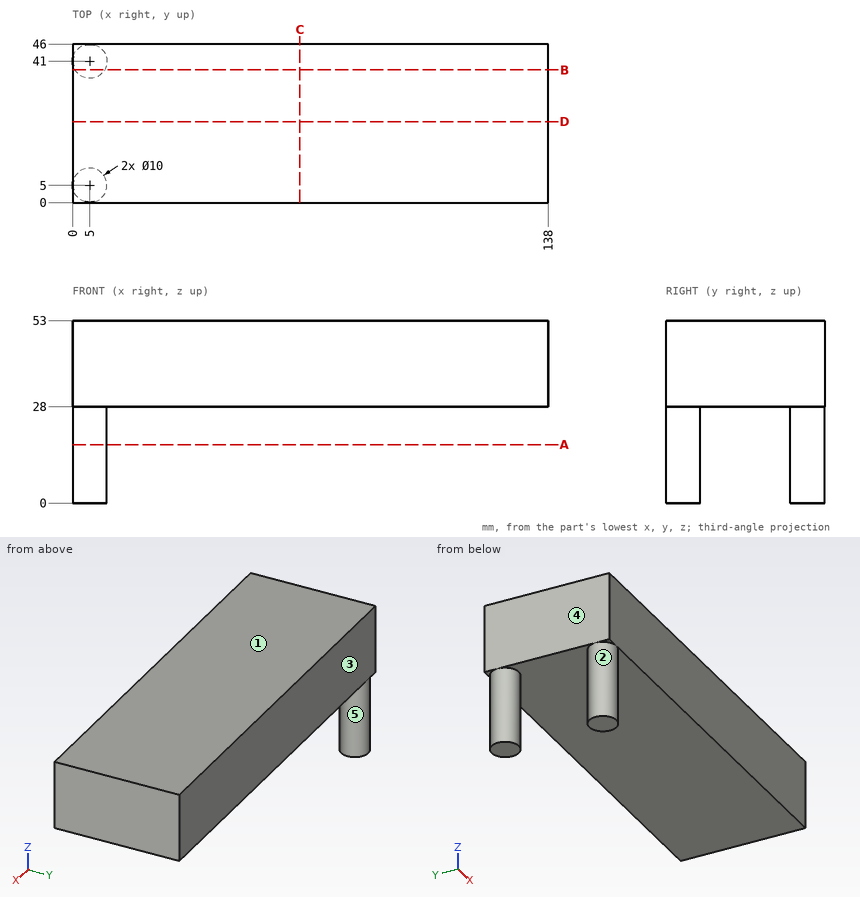
Check sheet for the drawn part. Datum: minimum x, y, z corner. Units: mm. A direction names the side the tool comes from. Round coordinates to 2 decimals unless told otherwise and drop trailing zeros. Write each loop counter-clockwise with the first axis right and the second up, starting at its lowest first coordinate (ties: lowest second). Pieces come first, ordered by that corner, then holes. Notation, with made-up numbers: (54.25, -15.75) - (83.25, -15.75) arc R15 cw to (83.25, -3.75) - close; hole circle Ø2 at (7, 27). An arc over 180 degrees is marked (long way). Return JSON: item names as keys, results as strings.
Q1. Depth check by flat-ended pin: P1, Ø1.5, axis at x = 46.5, z = 32.5, coming from the -Y side; P2, Ø14, axis at x = 50, y = 18.5, coming from the -Z side. Enter the tip coordinate at first touch or a pass-through.
Returned:
{"P1": "stops at y = 0", "P2": "stops at z = 28"}
Q2. Cross-section at C-C (x = 66). Record the boundary of the cut face in (y, z), then the cut area to 3 significant figures.
Returned:
{"outline": "(0, 28) - (46, 28) - (46, 53) - (0, 53) - close", "area": "1,150 mm²"}
Q3. Cross-section at A-A (z = 17). Record the boundary of the cut face in (x, y).
Returned:
{"outline": "circle Ø10 at (5, 5); circle Ø10 at (5, 41)"}
Q4. Draft check along Y on the marked faces 1, 2 and 3. Enter one of: released by +Y, released by -Y, zero draft, split by the parting line, or undercut.
Returned:
{"face 1": "zero draft", "face 2": "undercut", "face 3": "released by +Y"}
Q5. Access from +Z, -Z, +X, -X, +Y, -Y to the whole of each face (thin tool, end or side, straight path). Record for the marked faces 4 and 5.
Returned:
{"face 4": "+Z, -Z, -X, +Y, -Y", "face 5": "-Z"}
Q6. Scan lines: L1, parallel to Z at x = 114.5, y = 25; L2, parallel to X at y = 5.5, z = 9; L3, parallel to X at y = 37, z = 26.5. Record each from-to range of solid material in increasing order. Write a range as from..to.
Returned:
{"L1": "z = 28..53", "L2": "x = 0.03..9.97", "L3": "x = 2..8"}
Q7. Cross-section at B-B (y = 38.5). Record the boundary of the cut face in (x, z).
Returned:
{"outline": "(0, 28) - (0.67, 28) - (0.67, 0) - (9.33, 0) - (9.33, 28) - (138, 28) - (138, 53) - (0, 53) - close"}
Q8. Cross-section at D-D (y = 23.5). Record the boundary of the cut face in (x, z).
Returned:
{"outline": "(0, 28) - (138, 28) - (138, 53) - (0, 53) - close"}
